Check sheet for the modelled part. Datum: model origin and axes. Units: mm. A direction names the side the tool comes from. Give positions to 0.01 mm unless a question says otherwise; leave off trailing zeros. Order: outer loops, then holes, each group sorted by start corner. A loop starts at its lowest first (then second) coordinate and runs counter-clockwise, first axis right, second up.
Solid Edge part; units mm, degrees
sketch "Sketch1" plane through (0, 0, 0) normal (0, 0, 1) x (1, 0, 0)
  circle A0 centre (0, 0) radius 5
extrude "Protrusion1" add sketch "Sketch1" along normal blind 6
sketch "Sketch2" plane through (0, 0, 0) normal (0, 0, -1) x (1, 0, 0)
  circle A0 centre (0, 0) radius 3
extrude "Protrusion2" add sketch "Sketch2" along normal blind 75
sketch "Sketch3" plane through (0, 0, -75) normal (0, 0, -1) x (1, 0, 0)
  circle A0 centre (0, 0) radius 2.9997
extrude "Cutout1" cut sketch "Sketch3" against normal blind 24 flip side to cut
chamfer "Chamfer_1" distance 0.45 angle 45 1 edges at (-2.9997, 0, -75)
sketch "Sketch4" plane through (0, 0, 6) normal (0, 0, 1) x (1, 0, 0)
  line L0 (-1.4434, 2.5) -> (1.4434, 2.5)
  line L1 (2.8868, 0) -> (1.4434, 2.5)
  line L2 (1.4434, -2.5) -> (2.8868, 0)
  line L3 (-1.4434, -2.5) -> (1.4434, -2.5)
  line L4 (-2.8868, 0) -> (-1.4434, -2.5)
  line L5 (-1.4434, 2.5) -> (-2.8868, 0)
extrude "Cutout2" cut sketch "Sketch4" against normal blind 3
properties part number "185713" material "Stainless Steel, 304"
(1) Material ranges on L1, parallel to Z at x = 4.75, y = -1; L2, parallel to Y at x = -0.25, z = -68; L3, parallel to X at y = 2.25, z = -15, recorded low to high.
Response values:
L1: z = 0 to 6
L2: y = -2.99 to 2.99
L3: x = -1.98 to 1.98
(2) Gauge pin test, flat ends, axial feed: pin 1 Ø1.5 at (y, z) = (-3, -29) entering from -X; pin 2 Ø4 at (y, z) = (4, -39.5) entering from -X; pin 3 Ø4 at (y, z) = (0.5, -29.5) entering from -X. Record the tip position at first contact, or that the pin passes through.
Response values:
pin 1: stops at x = -1.98
pin 2: stops at x = -2.24
pin 3: stops at x = -3
(3) Set-up check for faces 1 (the face through (-1.08, 4.88, 2.96)), 2 (the face through (-2.155, 1.267, 4.521)), 3 (the face through (3.3, 0.1, 0)): record each of +Z, -Z, +X, -X, +Y, -Y from which the full face is reachable in a straight line by a thin tool's end or side.
Response values:
face 1: +Z, -Z
face 2: +Z
face 3: -Z
(4) Cross-section at B-B on z = -58. Enter the section's corners in (x, y), then the cut area to 3 significant figures.
Response values:
outline: circle Ø6 at (0, 0)
area: 28.3 mm2
(5) Cross-section at C-C on y = 4.25. Enter the section's corners in (x, z), then the cut area to 3 significant figures.
Response values:
outline: (-2.63, 0) - (2.63, 0) - (2.63, 6) - (-2.63, 6) - close
area: 31.6 mm2
